Could you check a few things on this drawing? It's one solid part, dimensions in mm from its lowest x, y, z. A direction names the side the tool comes from. Round coordinates to 2 decimals unless told otherwise and drop trailing zeros. Order: outer loops, then holes, each group sorted by start corner. A loop starts at its lowest first (then second) coordinate and runs counter-clockwise, first axis right, second up. Notation, with made-up numbers: (52.5, 84) - (106.5, 84) arc R13 cw to (106.5, 107) - close; hole circle Ø5 at (4.5, -37). An arc over 180 degrees is marked (long way). Use one line per item in the form item = value.
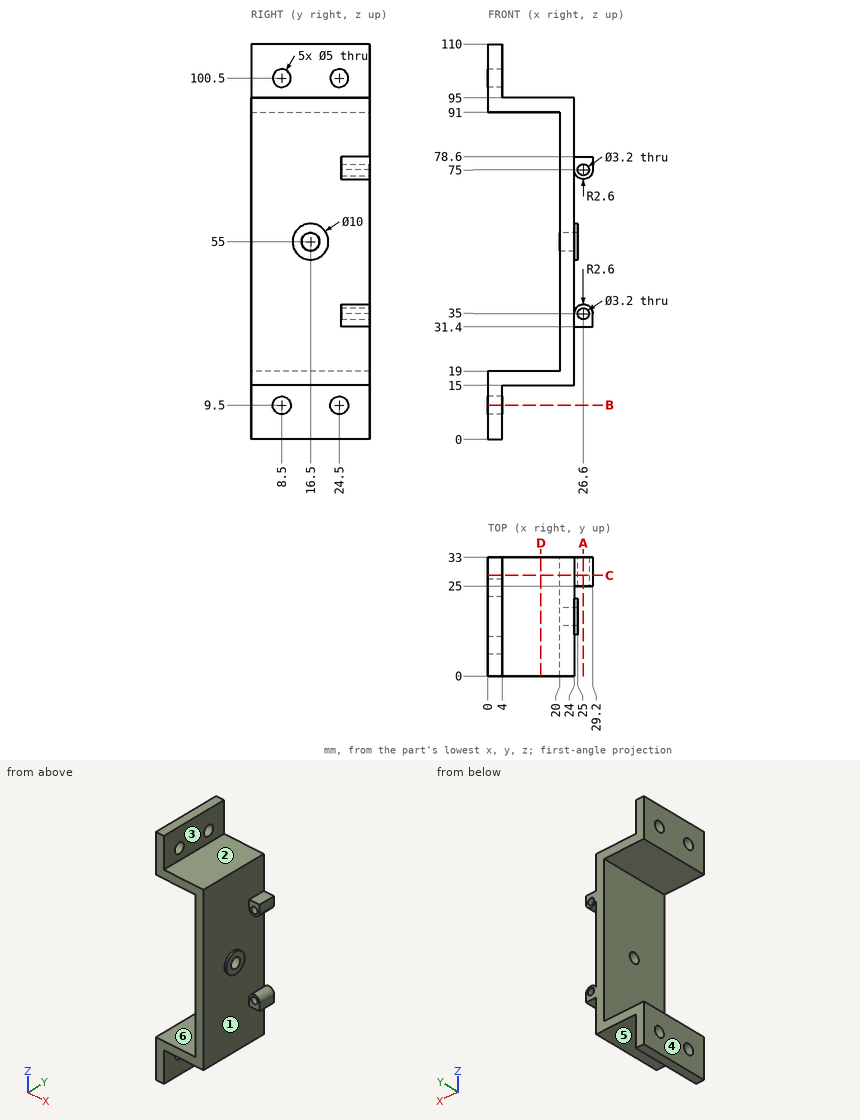
Item 1: Imagine slicing it at B-B on z = 9.5. Please give me the cut outline in (x, y), plus the area to 3 significant figures.
Found:
outline = (0, 0) - (4, 0) - (4, 6) - (0, 6) - close; (0, 11) - (4, 11) - (4, 22) - (0, 22) - close; (0, 27) - (4, 27) - (4, 33) - (0, 33) - close
area = 92.0 mm2
Item 2: Will these pins go through, and if not, where does the flat tip stop? P1, Ø8, axis at y = 24.5, z = 100.5, coming from the +X side; P2, Ø5, axis at y = 14, z = 46.5, coming from the -X side; P3, Ø5, axis at y = 9, z = 57, coming from the +X side; P4, Ø4.5, axis at y = 24.5, z = 9.5, coming from the -X side.
Found:
P1 = 4
P2 = 20
P3 = 24
P4 = through
Item 3: Imagine slicing it at A-A on x = 26.6. Please give me the cut outline in (y, z), plus the area to 3 significant figures.
Found:
outline = (25, 31.4) - (33, 31.4) - (33, 33.4) - (25, 33.4) - close; (25, 36.6) - (33, 36.6) - (33, 37.6) - (25, 37.6) - close; (25, 72.4) - (33, 72.4) - (33, 73.4) - (25, 73.4) - close; (25, 76.6) - (33, 76.6) - (33, 78.6) - (25, 78.6) - close
area = 48.0 mm2
Item 4: I need wall thicknesses on L1, parallel to Z at x = 26.6, y = 28.75; L2, parallel to Y at x = 2.5, z = 9.5; L3, parallel to Z at x = 1.05, y = 24.5. Which ranges of each line are inside material? Lowest first, please.
Found:
L1 = 31.4 to 33.4, 36.6 to 37.6, 72.4 to 73.4, 76.6 to 78.6
L2 = 0 to 6, 11 to 22, 27 to 33
L3 = 0 to 7, 12 to 19, 91 to 98, 103 to 110
Item 5: Imagine slicing it at C-C on y = 28. Please give me the cut outline in (x, z), plus the area to 3 significant figures.
Found:
outline = (0, 0) - (4, 0) - (4, 15) - (24, 15) - (24, 31.4) - (29.2, 31.4) - (29.2, 35) arc R2.6 ccw to (24, 35) - (24, 75) arc R2.6 ccw to (29.2, 75) - (29.2, 78.6) - (24, 78.6) - (24, 95) - (4, 95) - (4, 110) - (0, 110) - (0, 91) - (20, 91) - (20, 19) - (0, 19) - close; hole circle Ø3.2 at (26.6, 35); hole circle Ø3.2 at (26.6, 75)
area = 643 mm2
Item 6: Imagine slicing it at D-D on x = 14.75. Please give me the cut outline in (y, z), plus the area to 3 significant figures.
Found:
outline = (0, 15) - (33, 15) - (33, 19) - (0, 19) - close; (0, 91) - (33, 91) - (33, 95) - (0, 95) - close
area = 264 mm2
Item 7: For the marked faces 4, 5 and 6, which set-ups out of +Z, -Z, +X, -X, +Y, -Y let a thin tool reach every point of the face, with its end or its side?
Found:
face_4 = +Z, -Z, -X, +Y, -Y
face_5 = -Z, +X, +Y, -Y
face_6 = -X, +Y, -Y
Item 8: If we mould it in two halves opening along Z, with no side actions, what happens to the marked faces 1, 2 and 3? For each: released by +Z, released by -Z, zero draft, split by the parting line, or undercut.
Found:
face_1 = undercut
face_2 = released by +Z
face_3 = zero draft
